Verification items for this drawing (mm, ordinates from the low corner). A direction names the side the tool comes from. Give positions to 0.01 mm unless a question says otherwise; leave off trailing zeros. Loops run counter-clockwise (first coordinate to the right, second up) from the corner with the lowest first, then second, coordinate; pieces in that order, holes last. Notation, with made-up numbers: M 64,26.5 L 89,26.5 A7 ccw 89,33.5 Z; hole C 43,-18 d8. An arc over 180 degrees is marked long. Use one line per item in the form item = value.
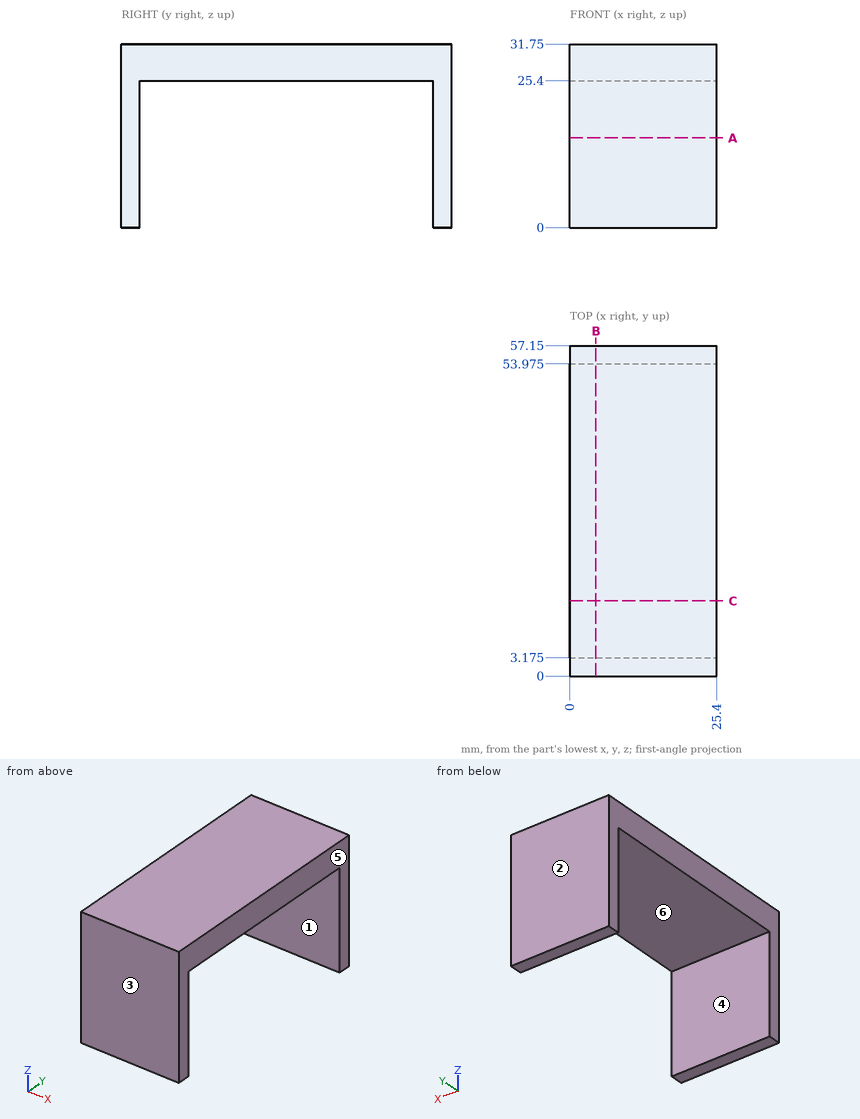
1) Section check A-A (z = 15.5). Record the cut outline in (x, y) (3 decimals), then the cut area to 3 significant figures.
Evaluation:
outline = M 0,0 L 25.4,0 L 25.4,3.175 L 0,3.175 Z; M 0,53.975 L 25.4,53.975 L 25.4,57.15 L 0,57.15 Z
area = 161 mm^2
2) Section check B-B (x = 4.5). Record the cut outline in (y, z) (3 decimals), then the cut area to 3 significant figures.
Evaluation:
outline = M 0,0 L 3.175,0 L 3.175,25.4 L 53.975,25.4 L 53.975,0 L 57.15,0 L 57.15,31.75 L 0,31.75 Z
area = 524 mm^2
3) Release check for a two-part mould opening along Y. For the marked faces 3, 4, 5 and 6 record: pulls with the +Y half, pulls with the -Y half, needs draft (parallel to the pull), parting line crosses it, or undercut.
Evaluation:
face_3 = pulls with the -Y half
face_4 = undercut
face_5 = needs draft
face_6 = undercut
4) Set-up check for the marked faces 1 and 2: record each of +Z, -Z, +X, -X, +Y, -Y from which the full face is reachable in a straight line by a thin tool's end or side.
Evaluation:
face_1 = -Z, +X, -X
face_2 = +Z, -Z, +X, -X, +Y
5) Scan lines: line 1 (Y direction, x = 20, z = 12.5) (3 decimals); line 2 (Z direction, x = 9, y = 35.5). Record each from-to range of solid material in increasing order.
Evaluation:
line_1 = 0 to 3.175, 53.975 to 57.15
line_2 = 25.4 to 31.75
6) Section check C-C (y = 13). Record the cut outline in (x, z), then the cut area to 3 significant figures.
Evaluation:
outline = M 0,25.4 L 25.4,25.4 L 25.4,31.75 L 0,31.75 Z
area = 161 mm^2
7) Depth check by flat-ended pin: pin 1 Ø12.5 at (x, y) = (15.5, 39.5) entering from -Z. Enter the tip coordinate at first touch or a pass-through.
Evaluation:
pin_1 = 25.4
